Can you work these out from the drawing? Everything is in mm from the part's minimum corner. Round coordinates to 2 decimals unless told otherwise and drop trailing zeros. Order: outer loops, then holes, each group sorted by start corner. A loop starts at its lowest first (then second) coordinate and runs counter-clockwise, first axis right, second up. Notation, with made-up numbers: (-1.75, -15.75) -> (17.25, -15.75) arc R24 cw to (17.25, 6.25) -> close; hole circle Ø5 at (-39.5, 12.5). An arc over 180 degrees is marked (long way). Use a Markdown table: item, result. Add a question column.
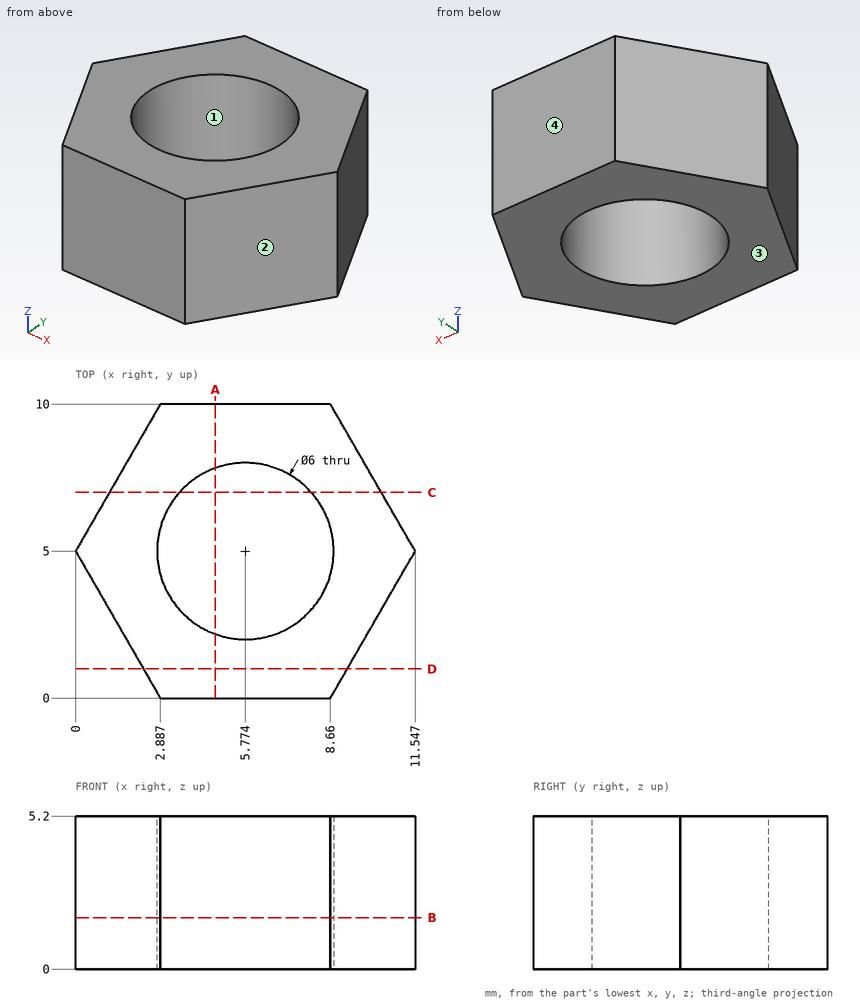
(1) I want a section at C-C on y = 7. List the corners of the cut face in (x, z) for me (1 decimal), and give its area (3 significant figures).
(2) If we mould it in two halves opening along Y, with no side actions, what happens to the marked faces 1, 2, 3 and 4? For each: pulls with the +Y half, pulls with the -Y half, needs draft (parallel to the pull), parting line crosses it, or undercut.
(3) I'm going to push a flat-ended pin straight in: P1, Ø3, axis at y = 2.5, z = 4, coming from the -X side. Where does the tip first touch, or does it pass through?
(4) I want a section at B-B on z = 1.75. List the corners of the cut face in (x, y) for me.
(5) Please list where these lines run through material, in increasing order: probe 1 along Y at (x, z) = (4, 0.8); probe 2 along X at (y, z) = (3.75, 1.8) (1 decimal); probe 3 along X at (y, z) = (6, 2.2) (1 decimal). Write a range as from..to.
(6) I want a section at A-A on x = 4.75. List the corners of the cut face in (y, z) for me.
(7) I want a section at D-D on y = 1. List the corners of the cut face in (x, z) for me.
Output:
| question | item | result |
|---|---|---|
| 1 | outline | (1.2, 0) -> (3.5, 0) -> (3.5, 5.2) -> (1.2, 5.2) -> close; (8, 0) -> (10.4, 0) -> (10.4, 5.2) -> (8, 5.2) -> close |
| 1 | area | 24.8 mm² |
| 2 | face 1 | undercut |
| 2 | face 2 | pulls with the -Y half |
| 2 | face 3 | needs draft |
| 2 | face 4 | pulls with the +Y half |
| 3 | P1 | x = 0.58 |
| 4 | outline | (0, 5) -> (2.89, 0) -> (8.66, 0) -> (11.55, 5) -> (8.66, 10) -> (2.89, 10) -> close; hole circle Ø6 at (5.77, 5) |
| 5 | probe 1 | 0..2.58, 7.42..10 |
| 5 | probe 2 | 0.7..3, 8.5..10.8 |
| 5 | probe 3 | 0.6..2.9, 8.6..11 |
| 6 | outline | (0, 0) -> (2.18, 0) -> (2.18, 5.2) -> (0, 5.2) -> close; (7.82, 0) -> (10, 0) -> (10, 5.2) -> (7.82, 5.2) -> close |
| 7 | outline | (2.31, 0) -> (9.24, 0) -> (9.24, 5.2) -> (2.31, 5.2) -> close |
